Here's how the part is built. I have some questions about the finished solid (model axes, mm). Give positions to 0.01 mm unless a question says otherwise; leave off trailing zeros. Order: outer loops, then holes, each group sorted by start corner. A loop starts at its lowest first (then second) coordinate and runs counter-clockwise, first axis right, second up. Notation, with made-up numbers: M 30,-37.5 L 36,-37.5 A30 cw 36,-7.5 Z; hole C -36.75,51 d9. An arc over 180 degrees is marked long. Use one line per item in the form item = value.
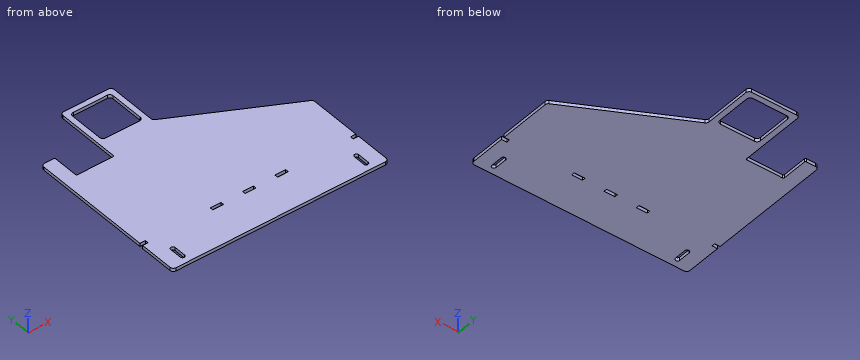
Autodesk Inventor part; units mm, degrees
ref_plane "YZ Plane" through (0, 0, 0) normal (1, 0, 0) x (0, 1, 0)
ref_plane "XZ Plane" through (0, 0, 0) normal (0, 1, 0) x (-1, 0, 0)
ref_plane "XY Plane" through (0, 0, 0) normal (0, 0, 1) x (1, 0, 0)
sketch "Boceto1" plane through (0, 0, 0) normal (0, 0, 1) x (1, 0, 0)
  line L0 (200, -200) -> (-200, -200)
  line L1 (-200, -200) -> (-200, 105)
  line L2 (-105, 105) -> (-105, 200)
  line L3 (-105, 200) -> (-10, 200)
  line L4 (-10, 200) -> (-10, 105)
  line L5 (200, -200) -> (200, -5)
  line L6 (200, -5) -> (-10, 105)
  line L7 (-20, 115) -> (-95, 115)
  line L8 (-95, 115) -> (-95, 190)
  line L9 (-95, 190) -> (-20, 190)
  line L10 (-20, 190) -> (-20, 115)
  line L11 (-20, 115) -> (-95, 190) construction
  line L12 (-95, 115) -> (-20, 190) construction
  line L13 (-200, 105) -> (-200, 125)
  line L14 (-200, 125) -> (-175, 125)
  line L15 (-175, 125) -> (-175, 75)
  line L16 (-175, 75) -> (-105, 75)
  line L17 (-105, 75) -> (-105, 105)
  point P0 (0, 0)
  point P1 (-57.5, 152.5)
  dimension "d0" = 305
  dimension "d1" = 95
  dimension "d2" = 95
  dimension "d3" = 195
  dimension "d4" = 400
  dimension "d7" = 75
  dimension "d8" = 75
  dimension "d9" = 20
  dimension "d10" = 25
  dimension "d11" = 50
extrude "Extrusión1" add sketch "Boceto1" along normal blind 6
fillet "Empalme1" radius 2 3 edges at (-175, 125, 3) (-175, 75, 3) (-105, 75, 3)
fillet "Empalme2" radius 6 11 edges at (-200, 125, 3) (-105, 200, 3) (-10, 200, 3) (-10, 105, 3) (-95, 115, 3) (-95, 190, 3) (-20, 190, 3) (-20, 115, 3) (200, -5, 3) (200, -200, 3) (-200, -200, 3)
sketch "Boceto2" plane through (0, 0, 6) normal (0, 0, 1) x (1, 0, 0)
  line L0 (10, -110) -> (-10, -110)
  line L1 (-10, -110) -> (-10, -104)
  line L2 (-10, -104) -> (10, -104)
  line L3 (10, -104) -> (10, -110)
  line L4 (10, -110) -> (-10, -104) construction
  line L5 (-10, -110) -> (10, -104) construction
  line L6 (-50, -110) -> (-70, -110)
  line L7 (-70, -110) -> (-70, -104)
  line L8 (-70, -104) -> (-50, -104)
  line L9 (-50, -104) -> (-50, -110)
  line L10 (-50, -110) -> (-70, -104) construction
  line L11 (-70, -110) -> (-50, -104) construction
  line L12 (70, -110) -> (50, -110)
  line L13 (50, -110) -> (50, -104)
  line L14 (50, -104) -> (70, -104)
  line L15 (70, -104) -> (70, -110)
  line L16 (70, -110) -> (50, -104) construction
  line L17 (50, -110) -> (70, -104) construction
  circle A0 centre (-170, -107) radius 4
  line L18 (-190, -110) -> (-210, -110)
  line L19 (-210, -110) -> (-210, -104)
  line L20 (-210, -104) -> (-190, -104)
  line L21 (-190, -104) -> (-190, -110)
  line L22 (-200, -149) -> (-200, 99)
  line L23 (-190, -110) -> (-210, -104) construction
  line L24 (-210, -110) -> (-190, -104) construction
  line L25 (0, 0) -> (0, -107)
  line L26 (210, -104) -> (190, -104)
  line L27 (190, -110) -> (210, -110)
  line L28 (190, -104) -> (190, -110)
  line L29 (210, -110) -> (210, -104)
  point P0 (-60, -107)
  point P1 (60, -107)
  point P2 (-200, -107)
  dimension "d16" = 20
  dimension "d17" = 6
  dimension "d18" = 20
  dimension "d19" = 60
  dimension "d20" = 20
  dimension "d21" = 60
  dimension "d22" = 8
  dimension "d23" = 20
  dimension "d24" = 6
  dimension "d25" = 110
  dimension "d27" = 6
  dimension "d28" = 6
  dimension "d29" = 107
extrude "Extrusión2" cut sketch "Boceto2" against normal through all contours L0 L1 L2 L3 | L6 L7 L8 L9 | L12 L13 L14 L15 | L18 L22 L20 L21 | L18 L19 L20 L22 | L29 L27 L28 L26
sketch "Boceto3" plane through (0, 0, 6) normal (0, 0, 1) x (1, 0, 0)
  line L0 (-194, -200) -> (194, -200)
  line L1 (0, -200) -> (0, -130)
  line L2 (0, -130) -> (-200, -130)
  line L3 (-200, -110) -> (-200, -194)
  line L4 (-200, -130) -> (-200, -120)
  line L5 (-200, -120) -> (200, -120)
  line L6 (200, -110) -> (200, -194)
  line L7 (0, -130) -> (200, -130)
  line L8 (200, -120) -> (200, -130)
  line L9 (10, -110) -> (-10, -110)
  line L10 (-10, -110) -> (-10, -104)
  line L11 (-10, -104) -> (10, -104)
  line L12 (10, -104) -> (10, -110)
  line L13 (10, -110) -> (-10, -104) construction
  line L14 (-10, -110) -> (10, -104) construction
  line L15 (-50, -110) -> (-70, -110)
  line L16 (-70, -110) -> (-70, -104)
  line L17 (-70, -104) -> (-50, -104)
  line L18 (-50, -104) -> (-50, -110)
  line L19 (-50, -110) -> (-70, -104) construction
  line L20 (-70, -110) -> (-50, -104) construction
  line L21 (70, -110) -> (50, -110)
  line L22 (50, -110) -> (50, -104)
  line L23 (50, -104) -> (70, -104)
  line L24 (70, -104) -> (70, -110)
  line L25 (70, -110) -> (50, -104) construction
  line L26 (50, -110) -> (70, -104) construction
  circle A0 centre (-170, -107) radius 4
  line L27 (-190, -110) -> (-210, -110)
  line L28 (-210, -110) -> (-210, -104)
  line L29 (-210, -104) -> (-190, -104)
  line L30 (-190, -104) -> (-190, -110)
  line L31 (-200, -149) -> (-200, 99)
  line L32 (-190, -110) -> (-210, -104) construction
  line L33 (-210, -110) -> (-190, -104) construction
  circle A1 centre (-80, -95) radius 3
  circle A2 centre (-80, -51) radius 3
  circle A3 centre (-170, -80) radius 3
  circle A4 centre (-170, -60) radius 3
  line L34 (0, 0) -> (0, -107)
  circle A5 centre (170, -107) radius 4
  line L35 (210, -104) -> (190, -104)
  line L36 (190, -110) -> (210, -110)
  line L37 (190, -104) -> (190, -110)
  line L38 (210, -110) -> (210, -104)
  circle A6 centre (80, -95) radius 3
  circle A7 centre (80, -51) radius 3
  circle A8 centre (170, -107) radius 13
  circle A9 centre (-170, -107) radius 13
  circle A10 centre (-170, -143) radius 13
  circle A11 centre (-170, -143) radius 4
  circle A12 centre (-170, -165) radius 4
  line L39 (-174, -143) -> (-174, -165)
  line L40 (-166, -165) -> (-166, -143)
  circle A13 centre (170, -143) radius 13
  circle A14 centre (170, -143) radius 4
  circle A15 centre (170, -165) radius 4
  line L41 (174, -143) -> (174, -165)
  line L42 (166, -165) -> (166, -143)
  point P0 (-60, -107)
  point P1 (60, -107)
  point P2 (-200, -107)
  dimension "d33" = 70
  dimension "d34" = 10
  dimension "d35" = 20
  dimension "d36" = 6
  dimension "d38" = 20
  dimension "d39" = 60
  dimension "d40" = 20
  dimension "d41" = 60
  dimension "d42" = 8
  dimension "d43" = 20
  dimension "d44" = 6
  dimension "d45" = 110
  dimension "d46" = 6
  dimension "d47" = 20
  dimension "d48" = 12
  dimension "d49" = 6
  dimension "d50" = 44
  dimension "d51" = 6
  dimension "d52" = 6
  dimension "d54" = 6
  dimension "d55" = 6
  dimension "d56" = 26
  dimension "d57" = 8
  dimension "d58" = 8
extrude "Extrusión3" cut sketch "Boceto3" against normal through all contours L39 A11 L40 A10 | A10 L40 A12 L39 | L42 A14 L41 A13 | A13 L41 A15 L42 | A11 | A12 | A15 | A14 picked at (-169.8393, -152.9432) picked at (170.1607, -152.9432)
sketch "Boceto5" plane through (0, 0, 6) normal (0, 0, 1) x (1, 0, 0)
  line L0 (-194, -200) -> (194, -200)
  line L1 (0, -200) -> (200, -200)
  line L2 (200, -200) -> (200, -180)
  line L3 (200, -194) -> (200, -110)
  line L4 (200, -180) -> (-200, -180)
  line L5 (-200, -110) -> (-200, -194)
  line L6 (-200, -200) -> (-200, -180)
  line L7 (-200, -200) -> (0, -200)
  point P0 (0, 0)
  dimension "d61" = 20
extrude "Extrusión4" cut sketch "Boceto5" against normal through all
fillet "Empalme3" radius 6 2 edges at (-200, -180, 3) (200, -180, 3)
properties part number "INTERNAL SIDE PLATE" material "Acero, carbono"
Q1. I want a section at B-B on y = 143. Write out the boundary of the cut face in (x, z), then the cut area to 3 significant figures.
Found:
outline = M -105,0 L -95,0 L -95,6 L -105,6 Z; M -20,0 L -10,0 L -10,6 L -20,6 Z
area = 120 mm²
Q2. I'm going to push flat-ended pins straight in: pin 1 Ø1.8 at (x, z) = (197.5, 2) entering from -Y; pin 2 Ø1.8 at (y, z) = (-106.5, 2) entering from +X; pin 3 Ø1.8 at (x, z) = (-3.5, 3.5) entering from +Y; pin 4 Ø3 at (x, y) = (16.5, -68) entering from -Z. Where does each tip first touch, or does it pass through?
Found:
pin_1 = -179.41
pin_2 = 190
pin_3 = 102.07
pin_4 = 0
Q3. I want a section at D-D on y = 48. Write out the boundary of the cut face in (x, z), then the cut area to 3 significant figures.
Found:
outline = M -200,0 L 98.82,0 L 98.82,6 L -200,6 Z
area = 1,790 mm²
Q4. I want a section at A-A on x = -36.5. Write out the boundary of the cut face in (y, z), then the cut area to 3 significant figures.
Found:
outline = M -180,0 L 115,0 L 115,6 L -180,6 Z; M 190,0 L 200,0 L 200,6 L 190,6 Z
area = 1,830 mm²
Q5. I need wall thicknesses on L1, parallel to X at y = 140, z = 2.1; L2, parallel to X at y = 123, z = 2.6; L3, parallel to Y at x = -32, z = 1.85. Which ranges of each line are inside material? Lowest first, please.
Found:
L1 = -105 to -95, -20 to -10
L2 = -198.47 to -175, -105 to -95, -20 to -10
L3 = -180 to 115, 190 to 200
Q6. I want a section at C-C on x = -148. Write out the boundary of the cut face in (y, z).
Found:
outline = M -180,0 L 75,0 L 75,6 L -180,6 Z
